```python
from build123d import *

# Parameters (mm, degrees)
BASE_FLANGE1_DEPTH           = 0.2
EDGE_FLANGE1_STRIP_W         = 1.2
EDGE_FLANGE1_STRIP_H         = 0.2
EDGE_FLANGE1_STRIP_CUT_DEPTH = 11.5
EDGE_FLANGE1_DEPTH           = 11.5
F_1_7_1_7_DIAMETER_HOLE1_D   = 1.7


# Sheet-metal steps are written as plain solids
with BuildPart() as part:
    # Sketch1 → Base-Flange1 (new body)
    with BuildSketch(Plane(origin=(0, 0, 0), x_dir=(1, 0, 0), z_dir=(0, 1, 0))):
        Polygon((5.75399352, 10.137943159), (-0.213435895, 10.137943159), (-4.873652989, 5.477726065), (3.258074995, -2.654001919), (8.5, 2.587923086), (8.5, 7.391936679), align=None)
    extrude(amount=-BASE_FLANGE1_DEPTH)

    # Edge-Flange1 strip (across the edge) → Edge-Flange1 strip cut (cut)
    with BuildSketch(Plane(origin=(3.258074995, -0.2, 2.654001919), x_dir=(0.707106781186555, -3.4914813388431337e-15, -0.70710678118654), z_dir=(-0.70710678118654, 0, -0.707106781186555))):
        with Locations((-0.4, -0.1)):
            Rectangle(EDGE_FLANGE1_STRIP_W, EDGE_FLANGE1_STRIP_H)
    extrude(amount=EDGE_FLANGE1_STRIP_CUT_DEPTH, mode=Mode.SUBTRACT)

    # Edge-Flange1 section (across the edge) → Edge-Flange1 (add)
    with BuildSketch(Plane(origin=(3.258074995, -0.2, 2.654001919), x_dir=(0.707106781186555, -3.4914813388431337e-15, -0.70710678118654), z_dir=(-0.70710678118654, 0, -0.707106781186555))):
        with BuildLine():
            Line((-0.2, 0.2), (-0.2, 0.8))
            Line((-0.2, 0.8), (0, 0.8))
            Line((0, 0.8), (0, 0.2))
            ThreePointArc((0, 0.2), (0.058578644, 0.058578644), (0.2, 0))
            Line((0.2, 0), (0.2, -0.2))
            ThreePointArc((0.2, -0.2), (-0.082842712, -0.082842712), (-0.2, 0.2))
        make_face()
    extrude(amount=EDGE_FLANGE1_DEPTH)

    # Ø1.7 (1.7) Diameter Hole1 (through all)
    with Locations(Plane(origin=(0, 0, 0), x_dir=(1, 0, 0), z_dir=(0, 1, 0))):
        with Locations((1.00251186, 7.818357007), (5.598705937, 3.22216293)):
            Hole(F_1_7_1_7_DIAMETER_HOLE1_D / 2)


solid = part.part
```
The listing builds one solid part. Answer for the finished solid, in the listing's coordinates (mm). A direction names the side the tool comes from. Give positions to 0.01 mm unless a question says otherwise; leave off trailing zeros. Order: outer loops, then holes, each group sorted by start corner. A loop starts at its lowest first (then second) coordinate and runs counter-clockwise, first axis right, second up. Notation, with made-up numbers: (-8.75, 57) - (0.25, 57) arc R26 ccw to (0.25, 86) - close; hole circle Ø5 at (14.25, -35.75). An arc over 180 degrees is marked (long way). Answer in a Markdown table with one row per item. Add a question column.
Q1. Find the intervals of material crossed by line 1 along Y through (x, z) = (1.5, -9.25); line 2 along Z through (x, y) = (-3.75, -0.3); line 3 along Z through (x, y) = (-2, -0.55), in increasing order. Write a range as [from, to].
Q2. The part is cut by section C-C (x = 7.5). Determine the outline of the cut face in (y, z), then the cut area to 3 significant figures.
Q3. The part is cut by section B-B (y = -0.6). Determine the outline of the cut face in (x, z).
Q4. Which of the six approach directions +Z, -Z, +X, -X, +Y, -Y give full straight-line access (tool end or side, diameter ignored) to faces 1 (the cylindrical face through (-0.807, -0.114, -1.299)), 2 (the flat face through (3, -0.2, -5))?
Q5. Given P1, Ø4, axis at x = 7, z = -0.5, coming from the -Y side, flat-ended and moving along its own axis, determine where the tip first touches the part or whether it passes through.
Q6. The part is cut by section A-A (x = 5). Determine the outline of the cut face in (y, z).
Determined:
| question | item | result |
|---|---|---|
| 1 | line 1 | y = [-0.2, 0] |
| 1 | line 2 | z = [-4.39, -4.09] |
| 1 | line 3 | z = [-2.6, -2.32] |
| 2 | outline | (-0.2, -8.39) - (0, -8.39) - (0, -1.59) - (-0.2, -1.59) - close |
| 2 | area | 1.36 mm² |
| 3 | outline | (-5.02, -5.34) - (-4.87, -5.48) - (3.26, 2.65) - (3.12, 2.8) - close |
| 4 | face 1 | +Z, -X, +Y |
| 4 | face 2 | -Z, +X, -Y |
| 5 | P1 | stops at y = -0.2 |
| 6 | outline | (-0.2, -10.14) - (0, -10.14) - (0, -3.83) - (-0.2, -3.83) - close; (-0.2, -2.62) - (0, -2.62) - (0, 0.91) - (-0.2, 0.91) - close |
